```python
from build123d import *
from OCP.BRepFilletAPI import BRepFilletAPI_MakeChamfer

# Parameters (mm, degrees)
SKETCH1_W           = 27
SKETCH1_H           = 76.5
BOSS_EXTRUDE1_DEPTH = 27
CUT_EXTRUDE3_DEPTH  = 84.171509545
CUT_EXTRUDE4_DEPTH  = 84.171509545
CUT_EXTRUDE5_DEPTH  = 74.5
CHAMFER1_SIZE       = 4
CHAMFER1_SIZE2      = 0.349954654
CHAMFER2_SIZE       = 4
CHAMFER2_SIZE2      = 0.349954654
CHAMFER3_SIZE       = 1


# Read off the part's stored shape, not the designer's step: Boss-Extrude2
with BuildPart() as part:
    # Sketch1 → Boss-Extrude1 (new body)
    with BuildSketch(Plane(origin=(0, 0, 0), x_dir=(1, 0, 0), z_dir=(0, 1, 0))):
        Rectangle(SKETCH1_W, SKETCH1_H)
    extrude(amount=BOSS_EXTRUDE1_DEPTH)

    # Boss-Extrude2 outline → Boss-Extrude2 (revolve)
    with BuildSketch(Plane.XZ.offset(-13.5)):
        Polygon((0, -38.25), (0, -39.25), (4.75, -39.25), (5.75, -38.25), align=None)
    revolve(axis=Axis((0, 13.5, 0), (0, 0, 1)))

    # Sketch6 → Cut-Extrude3 (cut, through all)
    with BuildSketch(Plane(origin=(0, 0, -39.25), x_dir=(-1, 0, 0), z_dir=(0, 0, -1))):
        with BuildLine():
            ThreePointArc((3.25, 13.5), (-1.656175974, 16.296351399), (-1.562049935, 10.65))
            Line((-1.562049935, 10.65), (1.562049935, 10.65))
            ThreePointArc((1.562049935, 10.65), (2.796351399, 11.843824026), (3.25, 13.5))
        make_face()
    extrude(amount=-CUT_EXTRUDE3_DEPTH, mode=Mode.SUBTRACT)

    # Sketch7 → Cut-Extrude4 (cut, through all)
    with BuildSketch(Plane.XY.offset(38.25)):
        Polygon((-11.328427125, 0), (-13.5, 2.171572875), (-13.5, 0), align=None)
        Polygon((-13.5, 27), (-13.5, 24.828427125), (-11.328427125, 27), align=None)
        Polygon((13.5, 27), (11.328427125, 27), (13.5, 24.828427125), align=None)
        Polygon((13.5, 2.171572875), (11.328427125, 0), (13.5, 0), align=None)
    extrude(amount=-CUT_EXTRUDE4_DEPTH, mode=Mode.SUBTRACT)

    # Sketch7<3> → Cut-Extrude5 (cut)
    with BuildSketch(Plane.XY.offset(38.25)):
        Polygon((-13.5, 2.171572875), (-11.328427125, 0), (-13.5, 0), align=None)
        Polygon((-11.5, 24), (-13.5, 24), (-13.5, 27), (13.5, 27), (13.5, 24), (11.5, 24), (11.5, 3), (10.5, 2), (-10.5, 2), (-11.5, 3), align=None)
        Polygon((11.328427125, 0), (13.5, 0), (13.5, 2.171572875), align=None)
        Polygon((-13.5, 21), (-13.5, 19), (-12.5, 20), align=None)
        Polygon((13.5, 19), (12.5, 20), (13.5, 21), align=None)
    extrude(amount=-CUT_EXTRUDE5_DEPTH, mode=Mode.SUBTRACT)

    # Chamfer1: one chamfer whose edges measure the first distance from different faces: ONE call of the kernel's chamfer builder (chamfer() names one face for all edges)
    chamfer1_edges_1 = [part.edges().sort_by_distance(p)[0] for p in [
        (-13, 19.5, 38.25),
    ]]
    chamfer1_side_1 = [part.faces().sort_by_distance(p)[0] for p in [
        (-13, 19.5, 1),
    ]]
    chamfer1_edges_2 = [part.edges().sort_by_distance(p)[0] for p in [
        (-13, 20.5, 38.25),
    ]]
    chamfer1_side_2 = [part.faces().sort_by_distance(p)[0] for p in [
        (-13, 20.5, 1),
    ]]
    chamfer1 = BRepFilletAPI_MakeChamfer(part.part.solid().wrapped)
    for e in chamfer1_edges_1:
        chamfer1.Add(CHAMFER1_SIZE, CHAMFER1_SIZE2, e.wrapped, chamfer1_side_1[0].wrapped)  # the first distance lies on this face
    for e in chamfer1_edges_2:
        chamfer1.Add(CHAMFER1_SIZE, CHAMFER1_SIZE2, e.wrapped, chamfer1_side_2[0].wrapped)  # the first distance lies on this face
    add(Compound.cast(chamfer1.Shape()), mode=Mode.REPLACE)

    # Chamfer2: one chamfer whose edges measure the first distance from different faces: ONE call of the kernel's chamfer builder (chamfer() names one face for all edges)
    chamfer2_edges_1 = [part.edges().sort_by_distance(p)[0] for p in [
        (13, 19.5, 38.25),
    ]]
    chamfer2_side_1 = [part.faces().sort_by_distance(p)[0] for p in [
        (13, 19.5, 1),
    ]]
    chamfer2_edges_2 = [part.edges().sort_by_distance(p)[0] for p in [
        (13, 20.5, 38.25),
    ]]
    chamfer2_side_2 = [part.faces().sort_by_distance(p)[0] for p in [
        (13, 20.5, 1),
    ]]
    chamfer2 = BRepFilletAPI_MakeChamfer(part.part.solid().wrapped)
    for e in chamfer2_edges_1:
        chamfer2.Add(CHAMFER2_SIZE, CHAMFER2_SIZE2, e.wrapped, chamfer2_side_1[0].wrapped)  # the first distance lies on this face
    for e in chamfer2_edges_2:
        chamfer2.Add(CHAMFER2_SIZE, CHAMFER2_SIZE2, e.wrapped, chamfer2_side_2[0].wrapped)  # the first distance lies on this face
    add(Compound.cast(chamfer2.Shape()), mode=Mode.REPLACE)

    # Chamfer3
    chamfer3_edges = [part.edges().sort_by_distance(p)[0] for p in [
        (12.5, 24, -36.25),
        (-12.5, 24, -36.25),
    ]]
    chamfer(chamfer3_edges, length=CHAMFER3_SIZE)


solid = part.part
```
Build history of the part. All positions in model axes, mm. A direction names the side the tool comes from. Round coordinates to 2 decimals unless told otherwise and drop trailing zeros. Write each loop counter-clockwise with the first axis right and the second up, starting at its lowest first coordinate (ties: lowest second). Pieces come first, ordered by that corner, then holes.
1) Band-saw the part on B-B, the plane y = 6. List the corners of the cut face in (x, z), and give its area (3 significant figures).
2) Mould opens along Y. For faces 1 (the flat face through (-12.86, 20.61, 36.28)), 2 (the flat face through (0, 0, -1)), 3 (the flat face through (-12, 24, 2)) say: +Y half, -Y half, draft (parallel to the pull), parting line (faces both ways), or undercut.
3) 3-axis set-ups, long thin cutter, end or side, ignore diameter. For faces 4 (the flat face through (-12.89, 19.36, 36.28)), 5 (the flat face through (13, 24, 2)), 6 (the flat face through (12.89, 19.36, 36.28)): which of +Z, -Z, +X, -X, +Y, -Y reach the whole face in a straight line?
4) Drill centre lines: probe 1 along X at (y, z) = (6, -21); probe 2 along X at (y, z) = (13.5, -38); probe 3 along Y at (x, z) = (0, -38). Where is each one in solid material? Low to high.
5) Band-saw the part on A-A, the plane x = 0. List the corners of the cut face in (y, z).
6) Band-saw the part on C-C, the plane z = -31. List the corners of the cut face in (x, y), and give its area (3 significant figures).
7) Pin check, flat tips, straight feed: pin 1 (10 mm diameter, centred on x = 8, y = 3.5, fed in from -Z); pin 2 (7.5 mm diameter, centred on x = 0, y = 13.5, fed in from +Z); pin 3 (1.6 mm diameter, centred on x = -12.5, z = 16.5, fed in from +Y). Stop position of each tip, or through.
Ans:
1. outline: (-13.5, -38.25) - (13.5, -38.25) - (13.5, 38.25) - (11.5, 38.25) - (11.5, -36.25) - (-11.5, -36.25) - (-11.5, 38.25) - (-13.5, 38.25) - close
1. area: 352 mm2
2. face 1: undercut
2. face 2: -Y half
2. face 3: +Y half
3. face 4: +Z, -X
3. face 5: +Z, +X, -X, +Y
3. face 6: +Z, +X
4. probe 1: x = -13.5 to -11.5, 11.5 to 13.5
4. probe 2: x = -13.5 to -3.25, 3.25 to 13.5
4. probe 3: y = 0 to 10.65, 16.75 to 27
5. outline: (0, -38.25) - (7.75, -38.25) - (8.75, -39.25) - (10.65, -39.25) - (10.65, -36.25) - (2, -36.25) - (2, 38.25) - (0, 38.25) - close; (16.75, -39.25) - (18.25, -39.25) - (19.25, -38.25) - (27, -38.25) - (27, -36.25) - (16.75, -36.25) - close
6. outline: (-13.5, 2.17) - (-11.33, 0) - (11.33, 0) - (13.5, 2.17) - (13.5, 19) - (12.5, 20) - (13.5, 21) - (13.5, 24) - (11.5, 24) - (11.5, 3) - (10.5, 2) - (-10.5, 2) - (-11.5, 3) - (-11.5, 24) - (-13.5, 24) - (-13.5, 21) - (-12.5, 20) - (-13.5, 19) - close
6. area: 136 mm2
7. pin 1: stops at z = -38.25
7. pin 2: stops at z = -36.25
7. pin 3: stops at y = 24
